from build123d import *

# Parameters (mm, degrees)
BOSS_EXTRUDE1_DEPTH = 76.2
CUT_EXTRUDE2_START  = -1.5875
CUT_EXTRUDE2_DEPTH  = 1.5875
CIRPATTERN10_COUNT  = 8


with BuildPart() as part:
    # Sketch2 → Boss-Extrude1 (new body)
    with BuildSketch(Plane.XY):
        with BuildLine():
            Line((0, 0), (29.160477546, -70.399620377))
            Line((29.160477546, -70.399620377), (29.160477546, -123.606903324))
            Line((29.160477546, -123.606903324), (29.160477546, -161.706903324))
            ThreePointArc((29.160477546, -161.706903324), (20.619571416, -182.326474739), (0, -190.86738087))
            Line((0, -190.86738087), (-50.8, -190.86738087))
            Line((-50.8, -190.86738087), (-50.8, -189.27988087))
            Line((-50.8, -189.27988087), (0, -189.27988087))
            ThreePointArc((0, -189.27988087), (19.4970394, -181.203942724), (27.572977546, -161.706903324))
            Line((27.572977546, -161.706903324), (27.572977546, -123.606903324))
            Line((27.572977546, -123.606903324), (27.572977546, -70.715393761))
            Line((27.572977546, -70.715393761), (0, -4.148337413))
            Line((0, -4.148337413), (-27.572977546, -70.715393761))
            Line((-27.572977546, -70.715393761), (-27.572977546, -123.606903324))
            Line((-27.572977546, -123.606903324), (-29.160477546, -123.606903324))
            Line((-29.160477546, -123.606903324), (-29.160477546, -70.399620377))
            Line((-29.160477546, -70.399620377), (0, 0))
        make_face()
    boss_extrude1 = extrude(amount=BOSS_EXTRUDE1_DEPTH)

    # Sketch5 → Cut-Extrude2 (cut)
    with BuildSketch(Plane.XZ.offset(190.86738087).offset(CUT_EXTRUDE2_START)):
        Polygon((-50.8, 76.2), (-30.48, 68.58), (-50.8, 60.96), (-30.48, 53.34), (-50.8, 45.72), (-30.48, 38.1), (-50.8, 30.48), (-30.48, 22.86), (-50.8, 15.24), (-30.48, 7.62), (-50.8, 0), (-53.34, 0), (-53.34, 76.2), align=None)
    cut_extrude2 = extrude(amount=CUT_EXTRUDE2_DEPTH, mode=Mode.SUBTRACT)

    # CirPattern10: Boss-Extrude1, Cut-Extrude2 ×8 about axis
    cirpattern10_axis = Axis((0, 0, 0), (0, 0, 1))
    add([boss_extrude1.rotate(cirpattern10_axis, i * 360 / CIRPATTERN10_COUNT) for i in range(1, CIRPATTERN10_COUNT)])
    add([cut_extrude2.rotate(cirpattern10_axis, i * 360 / CIRPATTERN10_COUNT) for i in range(1, CIRPATTERN10_COUNT)], mode=Mode.SUBTRACT)


solid = part.part
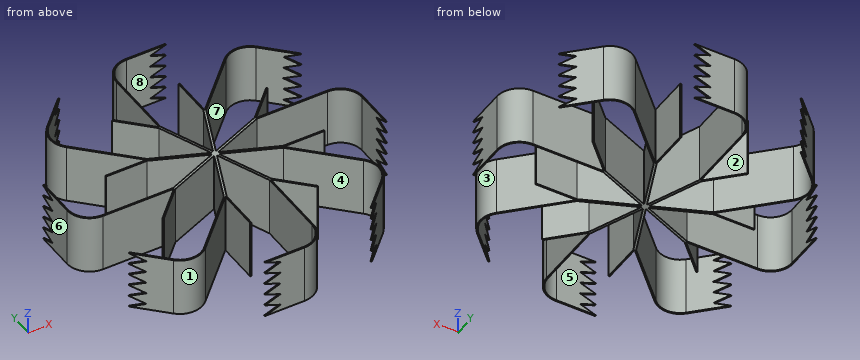
Can you work these out from the model? Positions are in its coordinate system, mm. Face numbers are marked on the shaded views. A direction names the side the tool comes from. Round coordinates to 2 decimals unless told otherwise and drop trailing zeros. Write each loop counter-clockwise with the first axis right and the second up, starting at its lowest first coordinate (ties: lowest second). Pieces come first, ordered by that corner, then holes. Notation, with made-up numbers: M 12.25,16.25 L 55.25,16.25 A14 cw 55.25,36.25 Z; hole C 86.5,-39 d7. An arc over 180 degrees is marked long. Use CSV: the item, a comma, the result in double quotes.
(1) I need wall thicknesses on line 1 along X through (y, z) = (-78, 40.5); line 2 along X through (y, z) = (2.5, 27); line 3 along X through (y, z) = (24, 21). Which ranges of each line are inside material? Lowest first, please.
Check values:
line 1,"-39.01 to -36.76, -29.16 to -27.57, 27.57 to 29.16, 36.76 to 39.01, 116.99 to 119.24"
line 2,"-190.87 to -189.28, -10.18 to 10.18, 189.17 to 190.76"
line 3,"-190.87 to -189.28, -62.09 to -53.79, -11.66 to -8.22, 8.22 to 11.66, 53.79 to 62.09, 175.28 to 178.27"
(2) Imagine slicing it at B-B (y = -148.5). Write out the boundary of the cut face in (x, z), plus the area to 3 significant figures.
Check values:
outline,"M 27.57,0 L 29.16,0 L 29.16,76.2 L 27.57,76.2 Z; M 119.18,0 L 121.43,0 L 121.43,76.2 L 119.18,76.2 Z"
area,"292 mm^2"
(3) On a 3-axis mill with a long thin cutter (end or side, diameter ignored), from which of +Z, -Z, +X, -X, +Y, -Y can I reach the whole of each face in a straight line? I mean the marked faces 1, 2, 3, 4 and 5. Say none if no direction works.
Check values:
face 1,"+Z, -Z, -Y"
face 2,"+Z, -Z, +Y"
face 3,"+Z, -Z, +X"
face 4,"+Z, -Z"
face 5,"+Z, -Z, -X"
(4) Imagine slicing it at D-D (x = 13.5). Write out the boundary of the cut face in (y, z).
Check values:
outline,"M -187.55,0 L -185.75,0 L -185.75,76.2 L -187.55,76.2 Z; M -36.74,0 L -28.44,0 L -28.44,76.2 L -36.74,76.2 Z; M -7.31,0 L -3.87,0 L -3.87,76.2 L -7.31,76.2 Z; M 3.87,0 L 7.31,0 L 7.31,76.2 L 3.87,76.2 Z; M 28.44,0 L 36.74,0 L 36.74,76.2 L 28.44,76.2 Z; M 189.28,0 L 190.87,0 L 190.87,76.2 L 189.28,76.2 Z"
(5) We'd pull the mould along X, two halves only. Please class the marked faces 6, 7 and 8: +X half, -X half, draft (parallel to the pull), parting line (faces both ways), or undercut.
Check values:
face 6,"-X half"
face 7,"undercut"
face 8,"draft"
(6) I'm going to push flat-ended pins straight in: pin 1 (2 mm diameter, centred on y = 120.5, z = 20.5, fed in from -X); pin 2 (1.5 mm diameter, centred on y = 38, z = 36, fed in from +X); pin 3 (3 mm diameter, centred on x = -26.5, z = 60.5, fed in from +Y). Where does each tip first touch, or does it pass through?
Check values:
pin 1,"x = -143.05"
pin 2,"x = 79.99"
pin 3,"y = 176.72"
(7) Imagine slicing it at A-A (x = 79). Write out the boundary of the cut face in (y, z).
Check values:
outline,"M -40.01,0 L -37.76,0 L -37.76,76.2 L -40.01,76.2 Z; M -29.16,0 L -27.57,0 L -27.57,76.2 L -29.16,76.2 Z; M 27.57,0 L 29.16,0 L 29.16,76.2 L 27.57,76.2 Z; M 37.76,0 L 40.01,0 L 40.01,76.2 L 37.76,76.2 Z; M 117.99,0 L 120.24,0 L 120.24,76.2 L 117.99,76.2 Z"
(8) Imagine slicing it at C-C (y = -84). Write out the boundary of the cut face in (x, z), plus the area to 3 significant figures.
Check values:
outline,"M -45.01,0 L -42.76,0 L -42.76,76.2 L -45.01,76.2 Z; M -29.16,0 L -27.57,0 L -27.57,76.2 L -29.16,76.2 Z; M 27.57,0 L 29.16,0 L 29.16,76.2 L 27.57,76.2 Z; M 42.76,0 L 45.01,0 L 45.01,76.2 L 42.76,76.2 Z; M 122.99,0 L 125.24,0 L 125.24,76.2 L 122.99,76.2 Z"
area,"755 mm^2"
